Autodesk Fusion 360 part; units mm, degrees
sketch "Sketch1" plane through (0, 0, 0) normal (1, 0, 0) x (0, 0, -1)
  circle A0 centre (0, 0) radius 2.575
  dimension "d1" = 5.15
extrude "Extrude1" add sketch "Sketch1" along normal blind 5
sketch "Sketch2" plane through (5, 0, 0) normal (1, 0, 0) x (0, 0, -1)
  circle A0 centre (0, 0) radius 2.575
  circle A1 centre (0, 0) radius 3.5
  dimension "d4" = 7
extrude "Extrude2" add sketch "Sketch2" along normal blind 2 contours A0 | A1
sketch "Sketch3" plane through (0, 0, 0) normal (1, 0, 0) x (0, 0, -1)
  circle A0 centre (0, 0) radius 1
  dimension "d7" = 2
extrude "Extrude3" cut sketch "Sketch3" along normal up to surface (7 mm away)
sketch "Sketch4" plane through (7, 0, 0) normal (1, 0, 0) x (0, 0, -1)
  circle A0 centre (0, 0) radius 1
  circle A1 centre (0, 0) radius 3.5
  line L0 (2.02, -2.1816) -> (-2.02, -2.1816) construction
  line L1 (-2.02, -2.1816) -> (-2.02, 2.1816) construction
  line L2 (-2.02, 2.1816) -> (2.02, 2.1816) construction
  line L3 (2.02, 2.1816) -> (2.02, -2.1816) construction
  line L4 (2.02, -2.1816) -> (-2.02, 2.1816) construction
  line L5 (-2.02, -2.1816) -> (2.02, 2.1816) construction
  line L6 (-2.02, 0) -> (2.02, 0) construction
  line L7 (0, -2.1816) -> (0, 2.1816) construction
  line L8 (-2.02, 1.137) -> (-2.02, -1.137)
  line L9 (2.02, 1.137) -> (2.02, -1.137)
  line L10 (-2.02, 1.137) -> (0, 2.1816)
  line L11 (0, 2.1816) -> (2.02, 1.137)
  line L12 (2.02, -1.137) -> (0, -2.1816)
  line L13 (0, -2.1816) -> (-2.02, -1.137)
  circle A2 centre (0, 0) radius 1.8654
  dimension "d10" = 4.04
  dimension "d11" = 4.3632
  dimension "d22" = 3.7308
fillet "Fillet1" radius 0.3 1 edges at (5, -0.9312, 2.4007)
fillet "Fillet2" radius 0.4 2 edges at (5, -1.2657, 3.2631) (7, -1.2657, 3.2631)
extrude "Extrude6" cut sketch "Sketch4" against normal blind 1.5804 contours A0 | A2
sketch "Sketch5" plane through (0, 0, 0) normal (1, 0, 0) x (0, 0, -1)
  line L0 (-3.5, 0) -> (3.5, 0)
  line L1 (3.5, 0) -> (3.5, -3.5)
  line L2 (3.5, -3.5) -> (-3.5, -3.5)
  line L3 (-3.5, -3.5) -> (-3.5, 0)
  dimension "d18" = 7
  dimension "d19" = 3.5
extrude "Extrude5" [suppressed]
equation "d1 = 5 mm * 1.03"
equation "d10 = ( 4 * 1.01 ) * 1 mm"
equation "d11 = ( 4.32 * 1.01 ) * 1 mm"
equation "d22 = 0.144 in * 1.02"
equation "d23 = -0.061 * 1.02 in"
Model file for the job. Use its own axes, mm. A direction names the side the tool comes from. Coordinates: 2 decimals unless noted, no trailing zeros. Write each loop counter-clockwise with the first axis right and the second up, starting at its lowest first coordinate (ties: lowest second). Pieces come first, ordered by that corner, then holes. Notation, with made-up numbers: (30, -31) -> (40, -31) arc R19 cw to (40, -5) -> close; hole circle Ø10 at (48.25, -4.5). An arc over 180 degrees is marked (long way). One line per item, written item: value. Start each with the question number.
1) Flat gauge pins, fed straight in: pin 1 Ø1 at (x, y) = (3, -2) entering from +Z; pin 2 Ø2.5 at (y, z) = (0, 0) entering from +X; pin 3 Ø1.9 at (y, z) = (1, -1) entering from +X; pin 4 Ø3 at (x, z) = (0.5, -1.5) entering from +Y (3 decimals). Where does each tip first touch, or does it go through?
2) Which spindle directions (+Z, -Z, +X, -X, +Y, -Y) get a long thin tool onto all of the face, cutting with end or side? Do faces 4 (the face through (2.317, -0.773, -2.456)), 5 (the face through (0, -1, -1)), 6 (the face through (6.221, 0.082, 1.864)). Say none if no direction does.
3) Pull direction Y, two halves, no side cores. Call faces 1 (the face through (5.42, -1, -1)), 2 (the face through (7, 0.04, -2.02)), 3 (the face through (5.992, 1.341, -3.233)): +Y half, -Y half, draft (parallel to the pull), parting line (faces both ways), or undercut.
4) Slice it at A-A on z = 0. Write the cut outline in (x, y) (3 decimals).
5) Slice it at C-C on x = 1. Write the cut outline in (y, z) (3 decimals).
6) Probe probe 1 along Y at (x, z) = (2.4, 0) (3 decimals); probe 2 along X at (y, z) = (-0.75, 0.75); probe 3 along X at (y, z) = (-1.75, 2.5). List the from-to ranges inside material, lowest first.
Answers follow:
1. pin 1: z = 2.09
1. pin 2: x = 5.42
1. pin 3: x = 7
1. pin 4: y = 2.575
2. face 4: -X
2. face 5: +Z, -Z, -X, +Y, -Y
2. face 6: +X
3. face 1: undercut
3. face 2: draft
3. face 3: parting line
4. outline: (0, -2.575) -> (4.7, -2.575) arc R0.3 cw to (5, -2.875) -> (5, -3.1) arc R0.4 ccw to (5.4, -3.5) -> (6.6, -3.5) arc R0.4 ccw to (7, -3.1) -> (7, -1.865) -> (5.42, -1.865) -> (5.42, -1) -> (0, -1) -> close; (0, 1) -> (5.42, 1) -> (5.42, 1.865) -> (7, 1.865) -> (7, 3.1) arc R0.4 ccw to (6.6, 3.5) -> (5.4, 3.5) arc R0.4 ccw to (5, 3.1) -> (5, 2.875) arc R0.3 cw to (4.7, 2.575) -> (0, 2.575) -> close
5. outline: circle Ø5.15 at (0, 0); hole circle Ø2 at (0, 0)
6. probe 1: -2.575 to -1, 1 to 2.575
6. probe 2: 0 to 5.42
6. probe 3: 5 to 7
